Read the model definition and answer for the solid it produces. Units are mm, in the model's axes. Coordinates: 2 decimals unless noted, no trailing zeros. Write each loop counter-clockwise with the first axis right and the second up, starting at its lowest first coordinate (ties: lowest second). Pieces come first, ordered by that corner, then holes.
Item 1: Each of these flat-tipped pins is pushed along its axis until it touches: P1, Ø5, axis at x = 38, z = 43, coming from the +Y side; P2, Ø1, axis at x = 88, z = 73, coming from the +Y side; P3, Ø4, axis at x = -8, z = 93.5, coming from the +Y side. Where does it stop, or does it pass through?
Item 2: Section B-B (z = 95.5) is taken. Give the vertices of the cut face in (x, y).
Item 3: Section A-A (x = -31) is taken. Give the vertices of the cut face in (y, z).
Item 4: Determine the mould class of faces 1 (the face through (2.8, 37.4, 64.2)), 2 (the face through (3, 39, 114.8)), 3 (the face through (88.2, 32.4, 16.3)), 4 (the face through (2.917, 39.897, 64.218)) for opening direction X: released by +X, released by -X, zero draft, split by the parting line, or undercut.
Item 5: Straight lines are drawn through the part: probe 1 along Y at (x, z) = (-14.5, 85.5); probe 2 along Y at (x, z) = (45, 101). For each, find the intervals that lie inside material, in ascending order.
from build123d import *

# Parameters (mm, degrees)
SKETCH005_W      = 295.497289
SKETCH005_H      = 102.6
SKETCH005_R      = 3.5
PAD005_DEPTH     = 2.5
HOLE_D           = 4.5
HOLE_DEPTH       = 25
HOLE_CSINK_D     = 13
HOLE_CSINK_ANGLE = 90


with BuildPart() as belt_backing_plate:
    # Sketch005 (on DatumPlane) → Pad005 (new body)
    with BuildSketch(Plane(origin=(2.415223, -39.927017, 0), x_dir=(0.998175, 0.060381, 0), z_dir=(0.060381, -0.998175, 0))):
        with Locations((2.570994, 63.5)):
            Rectangle(SKETCH005_W, SKETCH005_H)
        with Locations((-112, 107)):
            Circle(SKETCH005_R, mode=Mode.SUBTRACT)
        with Locations((-12, 107)):
            Circle(SKETCH005_R, mode=Mode.SUBTRACT)
        with Locations((88, 107)):
            Circle(SKETCH005_R, mode=Mode.SUBTRACT)
        with Locations((-112, 20)):
            Circle(SKETCH005_R, mode=Mode.SUBTRACT)
        with Locations((-12, 20)):
            Circle(SKETCH005_R, mode=Mode.SUBTRACT)
        with Locations((88, 20)):
            Circle(SKETCH005_R, mode=Mode.SUBTRACT)
    extrude(amount=-PAD005_DEPTH)

    # Hole
    with Locations(Plane(origin=(2.415223, -39.927017, 0), x_dir=(0.998175, 0.060381, 0), z_dir=(0.060381, -0.998175, 0))):
        with Locations((-112, 107), (-12, 107), (88, 107), (-112, 20), (-12, 20), (88, 20)):
            CounterSinkHole(HOLE_D / 2, HOLE_CSINK_D / 2, depth=HOLE_DEPTH, counter_sink_angle=HOLE_CSINK_ANGLE)


with BuildPart() as part_mirroring:
    # Part__Mirroring: instance of Belt backing plate
    add(belt_backing_plate.part.mirror(Plane(origin=(0, 0, 0), x_dir=(-1, 0, 0), z_dir=(0, -1, 0))))


solid = part_mirroring.part
Established:
1. P1: stops at y = 37.93
1. P2: stops at y = 34.78
1. P3: stops at y = 40.68
2. outline: (-142.65, 46.2) - (152.31, 28.36) - (152.46, 30.85) - (-142.5, 48.69) - close
3. outline: (39.44, 12.2) - (41.95, 12.2) - (41.95, 114.8) - (39.44, 114.8) - close
4. face 1: released by -X
4. face 2: zero draft
4. face 3: undercut
4. face 4: released by +X
5. probe 1: y = 38.45 to 40.95
5. probe 2: y = 34.85 to 37.35
